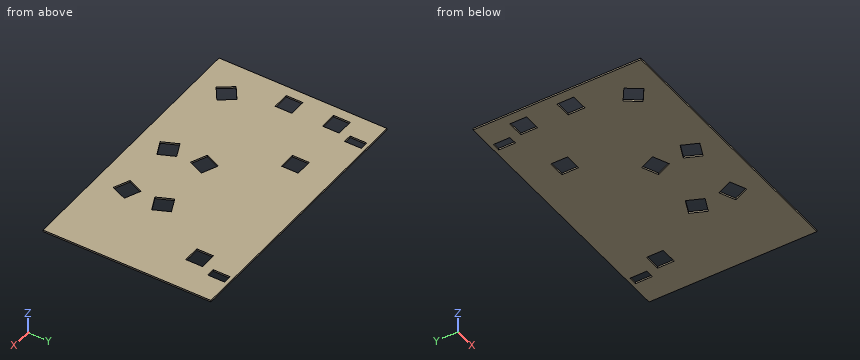
```python
from build123d import *

# Parameters (mm, degrees)
F0_W     = 203.2
F0_H     = 127
F0_W_2   = 12.7
F0_H_2   = 12.7
F0_W_3   = 6.35
F1_DEPTH = 1.27


with BuildPart() as f1:
    # F0 (on Top) → F1 (new body)
    with BuildSketch(Plane.XY):
        with Locations((-45.201082, 27.389223)):
            Rectangle(F0_W, F0_H)
        Polygon((-121.702438, -21.913276), (-129.066739, -11.566438), (-118.719901, -4.202136), (-111.355599, -14.548975), align=None, mode=Mode.SUBTRACT)
        Polygon((-50.755317, -5.224569), (-45.62584, -16.842592), (-57.243863, -21.972069), (-62.373341, -10.354046), align=None, mode=Mode.SUBTRACT)
        with Locations((-132.709693, 26.056859)):
            Rectangle(F0_W_2, F0_H_2, mode=Mode.SUBTRACT)
        Polygon((-57.243863, 21.972069), (-45.62584, 16.842592), (-50.755317, 5.224569), (-62.373341, 10.354046), align=None, mode=Mode.SUBTRACT)
        Polygon((-3.180643, -21.972069), (-14.798667, -16.842592), (-9.669189, -5.224569), (1.948834, -10.354046), align=None, mode=Mode.SUBTRACT)
        Polygon((-9.669189, 5.224569), (-14.798667, 16.842592), (-3.180643, 21.972069), (1.948834, 10.354046), align=None, mode=Mode.SUBTRACT)
        with Locations((-132.709693, 61.797474)):
            Rectangle(F0_W_2, F0_H_2, mode=Mode.SUBTRACT)
        with Locations((-124.576082, 81.781995)):
            Rectangle(F0_W_3, F0_H_2, mode=Mode.SUBTRACT)
        with Locations((-85.407068, 61.797474)):
            Rectangle(F0_W_2, F0_H_2, mode=Mode.SUBTRACT)
        with Locations((24.982561, 61.797474)):
            Rectangle(F0_W_2, F0_H_2, mode=Mode.SUBTRACT)
        with Locations((33.324402, 81.781995)):
            Rectangle(F0_W_3, F0_H_2, mode=Mode.SUBTRACT)
    extrude(amount=F1_DEPTH)


solid = f1.part
```
Check sheet for the modelled part. Datum: model origin and axes. Units: mm. Round coordinates to 2 decimals unless told otherwise and drop trailing zeros. Loops run counter-clockwise (first coordinate to the right, second up) from the corner with the lowest first, then second, coordinate; pieces in that order, holes last. Notation, with made-up numbers: (82, 3.5) -> (92, 3.5) arc R18 ccw to (92, 20.5) -> close; hole circle Ø5 at (-37, -36). An arc over 180 degrees is marked (long way). Answer in a Markdown table with one row per item.
Q1. Go/stop test with a flat-tipped pin: P1, Ø5, axis at x = 10, y = 72, coming from the -Z side. Record where the tip stops, or that it passes through.
Data:
| item | result |
|---|---|
| P1 | stops at z = 0 |
Q2. Thickness scan on L1, parallel to Y at x = -4.5, z = 0.1; L2, parallel to X at y = 25.5, z = 0.4; L3, parallel to Y at x = -14.5, z = 0.4. Record the ranges inside material, lowest first.
Data:
| item | result |
|---|---|
| L1 | y = -36.11 to -21.39, -7.51 to 7.51, 21.39 to 90.89 |
| L2 | x = -146.8 to -139.06, -126.36 to 56.4 |
| L3 | y = -36.11 to -16.97, -16.17 to 16.17, 16.97 to 90.89 |
Q3. Sectioned sample at B-B on y = 27.5. Enter the section's corners in (x, z).
Data:
| item | result |
|---|---|
| outline | (-146.8, 0) -> (-139.06, 0) -> (-139.06, 1.27) -> (-146.8, 1.27) -> close; (-126.36, 0) -> (56.4, 0) -> (56.4, 1.27) -> (-126.36, 1.27) -> close |
Q4. Sectioned sample at C-C on z = 0.2. Give the number of separate pieces and of enclosed holes in the cut face, then the cut area to 3 significant figures.
Data:
| item | result |
|---|---|
| separate pieces | 1 |
| enclosed holes | 11 |
| area | 24,200 mm^2 |
Q5. Sectioned sample at A-A on x = -82. Enter the section's corners in (y, z), then the cut area to 3 significant figures.
Data:
| item | result |
|---|---|
| outline | (-36.11, 0) -> (55.45, 0) -> (55.45, 1.27) -> (-36.11, 1.27) -> close; (68.15, 0) -> (90.89, 0) -> (90.89, 1.27) -> (68.15, 1.27) -> close |
| area | 145 mm^2 |
